Work out the finished part from the listing and answer in its coordinate system (mm). A direction names the side the tool comes from. Give positions to 0.01 mm unless a question says otherwise; leave off trailing zeros. Loops run counter-clockwise (first coordinate to the right, second up) from the corner with the lowest first, then second, coordinate; pieces in that order, holes last. Notation, with made-up numbers: (24, 8) -> (69, 8) arc R26 ccw to (69, 25) -> close; hole circle Ø6 at (34.5, -38). An arc over 180 degrees is marked (long way). Answer as CSV lines item,"result". Start each with the question number.
1. Find the intervals of material crossed by line 1 along X through (y, z) = (-4.5, -1); line 2 along Z through (x, y) = (-16.5, -5.25); line 3 along Z through (x, y) = (7.5, -7), in increasing order.
2. Determine the mould class of faces 3 (the face through (-131.269, -5, 49)), 4 (the face through (78.731, -5, 49)), 5 (the face through (-31.269, -5, 87)) for opening direction X: +X half, -X half, draft (parallel to the pull), parting line (faces both ways), or undercut.
3. Find section B-B, the plane z = 40.5. Give the vertices of the cut face in (x, y), and give its area (3 significant figures).
4. A flat-ended cylindrical pin translates along its axis: pin 1 Ø2 at (x, z) = (43.5, 45.5) entering from -Y. Find the tip coordinate at first contact, or state that the pin passes through.
5. Find section A-A, the plane y = -3. Give the vertices of the cut face in (x, z).
6. A tool of negligible diameter and unlimited length cuts with its end or side. For faces 1 (the face through (30.968, -5.07, 58.856)), 2 (the face through (75.724, -5.07, -21.913)), from which of +Z, -Z, +X, -X, +Y, -Y can it reach the whole face along a straight path? Write none if from no direction.
7. Find section C-C, the plane x = -4. Give the vertices of the cut face in (y, z).
from build123d import *

# Parameters (mm, degrees)
F0_W     = 210
F0_H     = 150
F1_DEPTH = 10
F2_R     = 10
F3_R     = 10
F4_R     = 10
F6_DEPTH = 10


with BuildPart() as f1:
    # F0 (on Front) → F1 (new body)
    with BuildSketch(Plane.XZ):
        with Locations((-26.2686859254, 50.2357134596)):
            Rectangle(F0_W, F0_H)
    extrude(amount=F1_DEPTH)

    # F2
    f2_edges = [f1.edges().sort_by_distance(p)[0] for p in [
        (-131.268686, -5, 125.235713),
    ]]
    fillet(f2_edges, radius=F2_R)

    # F3
    f3_edges = [f1.edges().sort_by_distance(p)[0] for p in [
        (-131.268686, -5, -24.764287),
    ]]
    fillet(f3_edges, radius=F3_R)

    # F4
    f4_edges = [f1.edges().sort_by_distance(p)[0] for p in [
        (78.731314, -5, -24.764287),
        (78.731314, -5, 125.235713),
    ]]
    fillet(f4_edges, radius=F4_R)

    # F5 (on face) → F6 (cut)
    with BuildSketch(Plane.XZ.offset(10)):
        with BuildLine():
            Line((-34.2686859254, -4.7642865404), (-31.2686859254, -4.7642865404))
            Line((-31.2686859254, -4.7642865404), (-31.2686859254, -1.7642865404))
            ThreePointArc((-31.2686859254, -1.7642865404), (-33.3900062689, -2.6429661969), (-34.2686859254, -4.7642865404))
        make_face()
        with BuildLine():
            Line((-31.2686859254, -7.7642865404), (-31.2686859254, -4.7642865404))
            Line((-31.2686859254, -4.7642865404), (-34.2686859254, -4.7642865404))
            ThreePointArc((-34.2686859254, -4.7642865404), (-33.3900062689, -6.885606884), (-31.2686859254, -7.7642865404))
        make_face()
        with BuildLine():
            Line((-31.2686859254, -4.7642865404), (-28.2686859254, -4.7642865404))
            ThreePointArc((-28.2686859254, -4.7642865404), (-29.1473655818, -2.6429661969), (-31.2686859254, -1.7642865404))
            Line((-31.2686859254, -1.7642865404), (-31.2686859254, -4.7642865404))
        make_face()
        with BuildLine():
            ThreePointArc((-31.2686859254, -7.7642865404), (-29.1473655818, -6.885606884), (-28.2686859254, -4.7642865404))
            Line((-28.2686859254, -4.7642865404), (-31.2686859254, -4.7642865404))
            Line((-31.2686859254, -4.7642865404), (-31.2686859254, -7.7642865404))
        make_face()
        with BuildLine():
            ThreePointArc((-31.2686859254, 66.2357134596), (18.9358955389, 45.4402949238), (39.7313140746, -4.7642865404))
            Line((39.7313140746, -4.7642865404), (42.7313140746, -4.7642865404))
            ThreePointArc((42.7313140746, -4.7642865404), (21.0572158824, 47.5616152674), (-31.2686859254, 69.2357134596))
            Line((-31.2686859254, 69.2357134596), (-31.2686859254, 66.2357134596))
        make_face()
        with BuildLine():
            ThreePointArc((-31.2686859254, 84.2357134596), (31.6638176002, 58.1682169852), (57.7313140746, -4.7642865404))
            Line((57.7313140746, -4.7642865404), (63.7313140746, -4.7642865404))
            ThreePointArc((63.7313140746, -4.7642865404), (35.9064582873, 62.4108576723), (-31.2686859254, 90.2357134596))
            Line((-31.2686859254, 90.2357134596), (-31.2686859254, 84.2357134596))
        make_face()
        with BuildLine():
            Line((-96.2686859254, 67.2357134596), (-96.2686859254, 73.2357134596))
            ThreePointArc((-96.2686859254, 73.2357134596), (-99.2686859254, 70.2357134596), (-96.2686859254, 67.2357134596))
        make_face()
        with BuildLine():
            ThreePointArc((-93.2686859254, 70.2357134596), (-94.1473655818, 72.3570338031), (-96.2686859254, 73.2357134596))
            Line((-96.2686859254, 73.2357134596), (-96.2686859254, 67.2357134596))
            ThreePointArc((-96.2686859254, 67.2357134596), (-94.1473655818, 68.114393116), (-93.2686859254, 70.2357134596))
        make_face()
        with BuildLine():
            ThreePointArc((-96.2686859254, 33.2357134596), (-99.2686859254, 30.2357134596), (-96.2686859254, 27.2357134596))
            Line((-96.2686859254, 27.2357134596), (-96.2686859254, 33.2357134596))
        make_face()
        with BuildLine():
            Line((-96.2686859254, 33.2357134596), (-96.2686859254, 27.2357134596))
            ThreePointArc((-96.2686859254, 27.2357134596), (-94.1473655818, 28.114393116), (-93.2686859254, 30.2357134596))
            ThreePointArc((-93.2686859254, 30.2357134596), (-94.1473655818, 32.3570338031), (-96.2686859254, 33.2357134596))
        make_face()
    extrude(amount=-F6_DEPTH, mode=Mode.SUBTRACT)


solid = f1.part
Resolved:
1,line 1,"x = -131.27 to 39.63, 42.64 to 57.65, 63.66 to 78.73"
1,line 2,"z = -24.76 to 64.68, 67.75 to 83, 89.08 to 125.24"
1,line 3,"z = -24.76 to 54.72, 58.27 to 75.35, 81.97 to 125.24"
2,face 3,"-X half"
2,face 4,"+X half"
2,face 5,"undercut"
3,outline,"(-131.27, -10) -> (23.43, -10) -> (23.43, 0) -> (-131.27, 0) -> close; (27.27, -10) -> (45.36, -10) -> (45.36, 0) -> (27.27, 0) -> close; (52.25, -10) -> (78.73, -10) -> (78.73, 0) -> (52.25, 0) -> close"
3,area,"1,990 mm^2"
4,pin 1,"passes through"
5,outline,"(-131.27, -14.76) arc R10 ccw to (-121.27, -24.76) -> (68.73, -24.76) arc R10 ccw to (78.73, -14.76) -> (78.73, 115.24) arc R10 ccw to (68.73, 125.24) -> (-121.27, 125.24) arc R10 ccw to (-131.27, 115.24) -> close; hole circle Ø6 at (-96.27, 30.24); hole circle Ø6 at (-96.27, 70.24); hole circle Ø6 at (-31.27, -4.76); hole (-31.27, 66.24) arc R71 cw to (39.73, -4.76) -> (42.73, -4.76) arc R74 ccw to (-31.27, 69.24) -> close; hole (-31.27, 84.24) arc R89 cw to (57.73, -4.76) -> (63.73, -4.76) arc R95 ccw to (-31.27, 90.24) -> close"
6,face 1,"+Y, -Y"
6,face 2,"-Z, +X, +Y, -Y"
7,outline,"(-10, -24.76) -> (0, -24.76) -> (0, 60.79) -> (-10, 60.79) -> close; (-10, 64.03) -> (0, 64.03) -> (0, 79.96) -> (-10, 79.96) -> close; (-10, 86.24) -> (0, 86.24) -> (0, 125.24) -> (-10, 125.24) -> close"
